Source: CAD feature listing. Evaluate the final solid. Frame: model axes, mm. Coordinates: 2 decimals unless noted, no trailing zeros. Write each loop counter-clockwise with the first axis right and the second up, starting at its lowest first coordinate (ties: lowest second). Pieces come first, ordered by that corner, then holes. Notation, with made-up numbers: (75.25, 67.5) -> (90.25, 67.5) arc R33 cw to (90.25, 106.5) -> close; hole circle Ø7 at (-1, -13.5). An arc over 180 degrees is marked (long way). Write item = value, one per line.
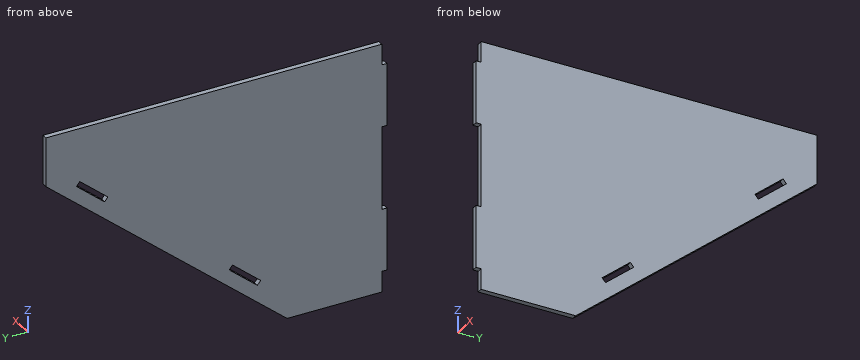
Autodesk Inventor part; units mm, degrees
ref_plane "YZ Plane" through (0, 0, 0) normal (1, 0, 0) x (0, 1, 0)
ref_plane "XZ Plane" through (0, 0, 0) normal (0, 1, 0) x (-1, 0, 0)
ref_plane "XY Plane" through (0, 0, 0) normal (0, 0, 1) x (1, 0, 0)
sketch "Sketch2" plane through (0, 0, 0) normal (1, 0, 0) x (0, 1, 0)
  line L0 (0, 0) -> (0, -12.7)
  line L1 (0, -12.7) -> (-3.175, -12.7)
  line L2 (-3.175, -12.7) -> (-3.175, -50.8)
  line L3 (-3.175, -50.8) -> (0, -50.8)
  line L4 (0, -50.8) -> (0, -101.6)
  line L5 (0, -101.6) -> (-3.175, -101.6)
  line L6 (-3.175, -101.6) -> (-3.175, -139.7)
  line L7 (-3.175, -139.7) -> (0, -139.7)
  line L8 (0, -139.7) -> (0, -152.4)
  line L9 (0, 0) -> (203.2, 0)
  line L10 (203.2, -29.949) -> (57.2685, -152.4)
  line L11 (203.2, -29.949) -> (203.2, 0)
  line L12 (0, -152.4) -> (57.2685, -152.4)
  dimension "d18" = 12.7
  dimension "d19" = 3.175
  dimension "d20" = 38.1
  dimension "d21" = 3.175
  dimension "d22" = 50.8
  dimension "d23" = 3.175
  dimension "d24" = 38.1
  dimension "d25" = 3.175
  dimension "d26" = 12.7
  dimension "d27" = 203.2
  dimension "d28" = 190.5
  dimension "d29" = 90
  dimension "d30" = -130
  dimension "d31" = 0
extrude "Extrusion2" add sketch "Sketch2" along normal blind 3.175
sketch "Sketch3" plane through (3.175, 0, 0) normal (1, 0, 0) x (0, 0, -1)
  line L0 (152.4, 57.2685) -> (29.949, 203.2)
  line L1 (152.4, 57.2685) -> (137.8069, 45.0234)
  line L2 (137.8069, 45.0234) -> (15.3558, 190.9549)
  line L3 (15.3558, 190.9549) -> (29.949, 203.2)
  line L4 (146.3195, 52.1664) -> (23.8685, 198.0979)
  line L5 (143.8873, 50.1256) -> (21.4363, 196.057)
  line L6 (32.661, 182.68) -> (35.0932, 184.7208)
  line L7 (46.9469, 165.6546) -> (49.3791, 167.6955)
  line L8 (110.2133, 90.2567) -> (112.6455, 92.2976)
  line L9 (124.4992, 73.2314) -> (126.9314, 75.2722)
  point P0 (0, 0)
  dimension "d34" = 19.05
  dimension "d35" = 3.175
  dimension "d36" = 7.9375
  dimension "d37" = 17.4625
  dimension "d38" = 22.225
  dimension "d39" = 98.425
  dimension "d40" = 22.225
extrude "Extrusion3" cut sketch "Sketch3" against normal blind 3.175 contours L9 L5 L8 L4 | L4 L7 L5 L6
properties part number "C4Side"
1) Material intervals for probe 1 along Z at (x, y) = (0.75, 75.5); probe 2 along Z at (x, y) = (1.9, 183); probe 3 along Y at (x, z) = (0.65, -46) (3 decimals), sorted ascending. Write a range as [from, to].
Answer block:
probe_1 = [-137.1, -126.74], [-122.6, 0]
probe_2 = [-46.9, -36.54], [-33.04, 0]
probe_3 = [-3.175, 166.783], [171.723, 184.071]
2) First-contact query: pin 1 Ø1 at (x, y) = (1, -2.5) entering from +Z; pin 2 Ø1 at (x, y) = (2, -2.5) entering from -Z; pin 3 Ø1.6 at (x, z) = (1, -72) entering from -Y. Flat tips, straight axial feed; report the tip coordinate or a pass-through.
Answer block:
pin_1 = -12.7
pin_2 = -139.7
pin_3 = 0
3) Cut plane C-C, the plane y = 156.5. Output: boundary loops of the cut face in (x, z) (3 decimals), and give its area (3 significant figures).
Answer block:
outline = (0, -69.135) -> (3.175, -69.135) -> (3.175, 0) -> (0, 0) -> close
area = 220 mm2
4) Cut plane B-B, the plane z = -88. Output: boundary loops of the cut face in (x, y) (3 decimals).
Answer block:
outline = (0, 0) -> (3.175, 0) -> (3.175, 134.017) -> (0, 134.017) -> close
5) Cut plane A-A, the plane x = 0.75. Output: boundary loops of the cut face in (y, z) (1 decimal).
Answer block:
outline = (-3.2, -139.7) -> (0, -139.7) -> (0, -152.4) -> (57.3, -152.4) -> (203.2, -29.9) -> (203.2, 0) -> (0, 0) -> (0, -12.7) -> (-3.2, -12.7) -> (-3.2, -50.8) -> (0, -50.8) -> (0, -101.6) -> (-3.2, -101.6) -> close; hole (73.2, -124.5) -> (75.3, -126.9) -> (92.3, -112.6) -> (90.3, -110.2) -> close; hole (165.7, -46.9) -> (167.7, -49.4) -> (184.7, -35.1) -> (182.7, -32.7) -> close
